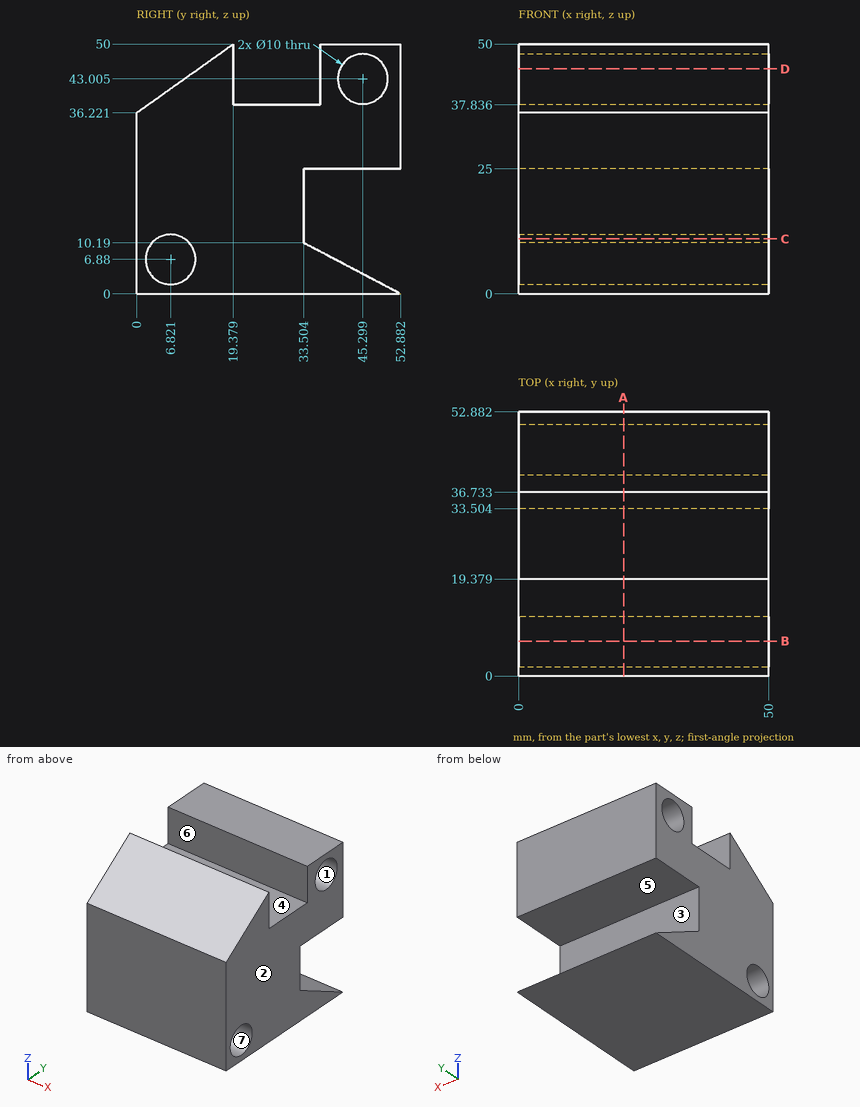
For this review, use the dimensioned drawing (mm, ordinates from the lowest corner) and the shaded views. A direction names the side the tool comes from. Coordinates: 2 decimals unless noted, no trailing zeros. Loops run counter-clockwise (first coordinate to the right, second up) from the corner with the lowest first, then second, coordinate; pieces in that order, holes last. Notation, with made-up numbers: (82, 78.25) -> (101, 78.25) arc R18 ccw to (101, 100.25) -> close; hole circle Ø9 at (-24.5, 78.5). An arc over 180 degrees is marked (long way). Return JSON: item names as keys, results as strings. Group by question number.
(1) Consider section D-D, the plane z = 45. Give the boundary of the cut face in (x, y) (1 decimal).
(2) Tool access review of the marked faces 5, 6 and 7: name each direction out of +Z, -Z, +X, -X, +Y, -Y from which nothing blocks a thin tool from reaching the whole face with its end or side.
(3) Consider section B-B, the plane y = 7. Give the boundary of the cut face in (x, z).
(4) Consider section C-C, the plane z = 11. Give the boundary of the cut face in (x, y), plus the area to 3 significant figures.
(5) To check wall thickness, follow L1, parallel to Y at x = 23, z = 38.5 (1 decimal); L2, parallel to Y at x = 11, z = 44.5 (1 decimal); L3, parallel to Z at x = 3, y = 23 (1 decimal). State the ranges of each line that lie inside material, in increasing order.
(6) For pin 1 Ø9.5 at (x, z) = (31.5, 44) entering from -Y; pin 2 Ø16.5 at (x, z) = (24.5, 19.5) entering from +Y; pin 3 Ø3 at (x, y) = (35.5, 33) entering from +Z; pin 4 Ø2 at (x, y) = (22, 18) entering from +Z, all flat-tipped, find the tip position at first contact; note any pin that passes through.
(7) Mouldability with a two-part tool opening along Z and no side actions: class the marked faces 1, 2, 3 and 4 as pulls with the +Z half, pulls with the -Z half, needs draft (parallel to the pull), parting line crosses it, or undercut.
(8) Consider section A-A, the plane x = 21. Give the boundary of the cut face in (y, z) (1 decimal), plus the area to 3 significant figures.
Results below:
{
 "1": {"outline": "(0, 12.3) -> (50, 12.3) -> (50, 19.4) -> (0, 19.4) -> close; (0, 36.7) -> (50, 36.7) -> (50, 40.7) -> (0, 40.7) -> close; (0, 49.9) -> (50, 49.9) -> (50, 52.9) -> (0, 52.9) -> close"},
 "2": {"face 5": "+X, -X, +Y", "face 6": "+Z, +X, -X", "face 7": "+X, -X"},
 "3": {"outline": "(0, 0) -> (50, 0) -> (50, 1.88) -> (0, 1.88) -> close; (0, 11.88) -> (50, 11.88) -> (50, 41.2) -> (0, 41.2) -> close"},
 "4": {"outline": "(0, 0) -> (50, 0) -> (50, 3.99) -> (0, 3.99) -> close; (0, 9.65) -> (50, 9.65) -> (50, 33.5) -> (0, 33.5) -> close", "area": "1,390 mm2"},
 "5": {"L1": "y = 3.2 to 19.4, 36.7 to 43.1, 47.5 to 52.9", "L2": "y = 11.6 to 19.4, 36.7 to 40.5, 50.1 to 52.9", "L3": "z = 0 to 37.8"},
 "6": {"pin 1": "stops at y = 4.26", "pin 2": "stops at y = 52.88", "pin 3": "stops at z = 37.84", "pin 4": "stops at z = 49.73"},
 "7": {"face 1": "undercut", "face 2": "needs draft", "face 3": "undercut", "face 4": "pulls with the +Z half"},
 "8": {"outline": "(0, 0) -> (52.9, 0) -> (33.5, 10.2) -> (33.5, 25) -> (52.9, 25) -> (52.9, 50) -> (36.7, 50) -> (36.7, 37.8) -> (19.4, 37.8) -> (19.4, 50) -> (0, 36.2) -> close; hole circle Ø10 at (6.8, 6.9); hole circle Ø10 at (45.3, 43)", "area": "1,760 mm2"}
}
